For this review, use the dimensioned drawing (mm, ordinates from the lowest corner) and the shaded views. A direction names the side the tool comes from. Coordinates: 2 decimals unless noted, no trailing zeros. Return JSON: item names as keys, results as strings. Group by question number.
Item 1: Draft analysis for pull direction Y (two halves, no side actions). For the marked faces 4, 5, 6 and 7, state which applies: +Y half, -Y half, draft (parallel to the pull), parting line (faces both ways), or undercut.
Item 2: Insertion check: pin 1 (0.9 mm diameter, centred on x = 2.5, z = 4, fed in from +Y) (1 decimal); pin 2 (1 mm diameter, centred on x = 2, y = 2, fed in from +Z) (1 decimal). Each pin has a flat end and moves straight along its axis. Give the tip position at first contact, or say it passes through.
Item 3: Machinability: for the marked faces 1, 2 and 3, which of the approach directions +Z, -Z, +X, -X, +Y, -Y give a long, thin tool a straight path to every point of the face, cutting with its end or side? Answer none if there is none.
Item 4: For line 1 along Z through (x, y) = (1.4, 1.25); line 2 along Y through (x, z) = (4, 5.5) (1 decimal); line 3 along Y through (x, z) = (1.6, 0.75), list the stretches that pass through material, from the lowest coordinate up.
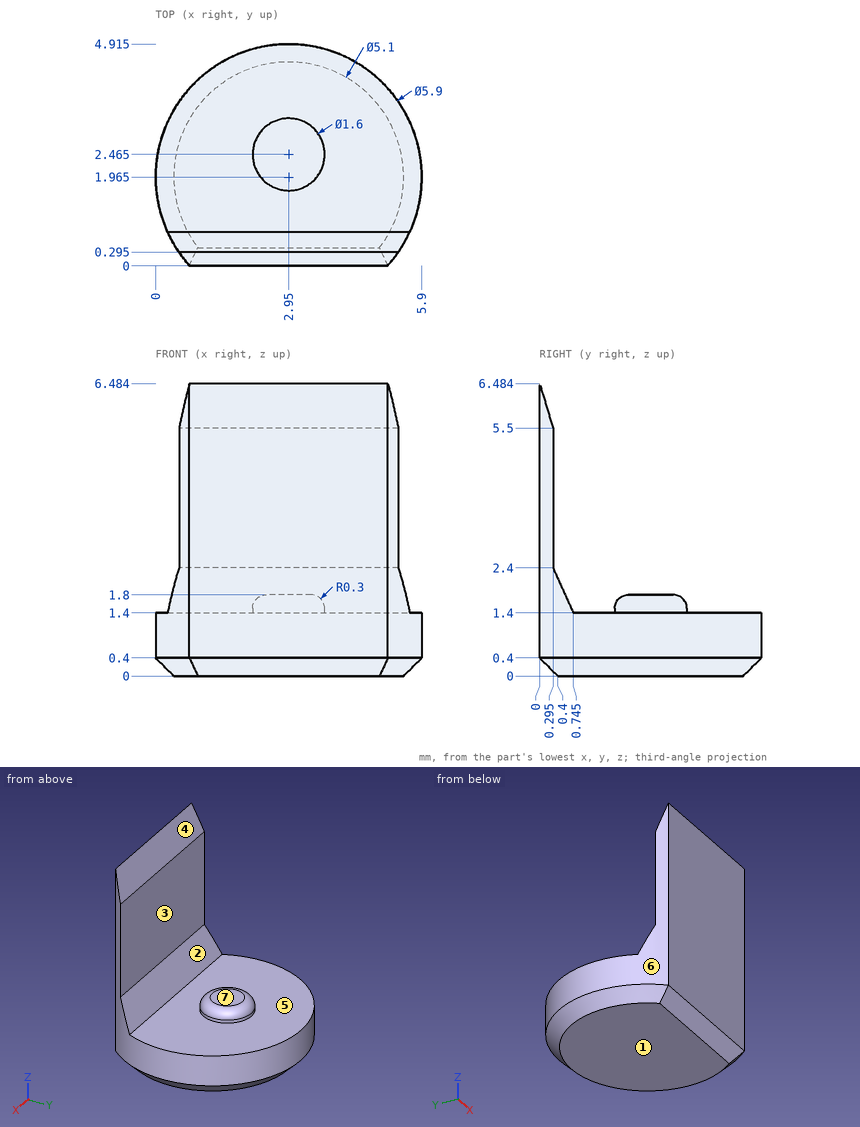
Findings below:
{
 "1": {"face 4": "+Y half", "face 5": "undercut", "face 6": "parting line", "face 7": "draft"},
 "2": {"pin 1": "stops at y = 0.3", "pin 2": "stops at z = 1.8"},
 "3": {"face 1": "-Z, +X, -X, +Y, -Y", "face 2": "+Z, +X, -X", "face 3": "+Z, +X, -X, +Y"},
 "4": {"line 1": "z = 0 to 1.4", "line 2": "y = 0 to 0.3", "line 3": "y = 0 to 4.59"}
}
